Read the model definition and answer for the solid it produces. Units are mm, in the model's axes. Face numbers are marked on the shaded views. A direction names the side the tool comes from. Coordinates: 2 decimals unless noted, no trailing zeros. Loops run counter-clockwise (first coordinate to the right, second up) from the corner with the lowest first, then second, coordinate; pieces in that order, holes last. Notation, with made-up numbers: M -33.75,67.5 L -3.75,67.5 A12 ccw -3.75,75.5 Z; hole C 20,26 d11. An arc over 180 degrees is marked long. Put each result on its own line as item: value.
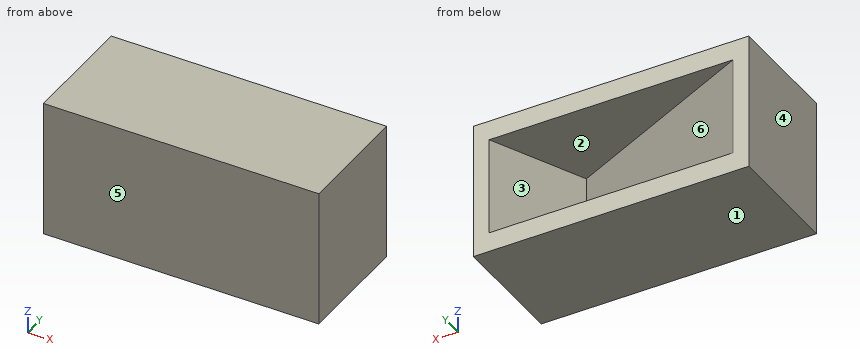
from build123d import *

# Parameters (mm, degrees)
SKETCH1_W           = 35
SKETCH1_H           = 17.5
BOSS_EXTRUDE2_DEPTH = 7.5
CUT_EXTRUDE2_DEPTH  = 6.25


with BuildPart() as part:
    # Sketch1 → Boss-Extrude2 (new, symmetric)
    with BuildSketch(Plane(origin=(0, 0, 0), x_dir=(1, 0, 0), z_dir=(0, 1, 0))):
        Rectangle(SKETCH1_W, SKETCH1_H)
    extrude(amount=BOSS_EXTRUDE2_DEPTH, both=True)

    # Sketch5 → Cut-Extrude2 (cut, symmetric)
    with BuildSketch(Plane.XY):
        Polygon((-15.5, 7.5), (9.96320795, -4.373688868), (15.5, 7.5), align=None)
    extrude(amount=CUT_EXTRUDE2_DEPTH, both=True, mode=Mode.SUBTRACT)


solid = part.part
1) Find section A-A, the plane y = 4.25. Write down the section's boundary in (x, z).
Answer list:
outline: M -17.5,-8.75 L 17.5,-8.75 L 17.5,8.75 L -17.5,8.75 Z; hole M -8.53,-6.25 L 13.98,-6.25 L 13.98,6.25 L -8.53,6.25 Z
2) Find section B-B, the plane x = -6. Write down the section's boundary in (y, z).
Answer list:
outline: M -7.5,-8.75 L 7.5,-8.75 L 7.5,-6.25 L 3.07,-6.25 L 3.07,6.25 L 7.5,6.25 L 7.5,8.75 L -7.5,8.75 Z
3) Find section D-D, the plane y = 2. Write down the section's boundary in (x, z).
Answer list:
outline: M -17.5,-8.75 L 17.5,-8.75 L 17.5,8.75 L -17.5,8.75 Z; hole M -3.71,-6.25 L 12.94,-6.25 L 12.94,6.25 L -3.71,6.25 Z
4) Find section C-C, the plane z = 1.5. Write down the section's boundary in (x, y), plus the area to 3 significant figures.
Answer list:
outline: M -17.5,-7.5 L 17.5,-7.5 L 17.5,7.5 L 15.5,7.5 L 9.96,-4.37 L -15.5,7.5 L -17.5,7.5 Z
area: 341 mm^2
5) Determine the mould class of the marked faces 1, 2, 3 and 4 for opening direction X: released by +X, released by -X, zero draft, split by the parting line, or undercut.
Answer list:
face 1: zero draft
face 2: undercut
face 3: undercut
face 4: released by -X
6) Which of the six approach directions +Z, -Z, +X, -X, +Y, -Y give full straight-line access (tool end or side, diameter ignored) to the marked faces 5 and 6?
Answer list:
face 5: +Z, -Z, +X, -X, -Y
face 6: +Y
7) Straight lines are drawn through the part: line 1 (Z direction, x = 8, y = -3.25); line 2 (X direction, y = 5.75, z = -1); line 3 (X direction, y = 1.5, z = -4). For each, find the intervals that lie inside material, in ascending order. Write a range as [from, to].
Answer list:
line 1: z = [-8.75, -6.25], [6.25, 8.75]
line 2: x = [-17.5, -11.75], [14.68, 17.5]
line 3: x = [-17.5, -2.63], [12.7, 17.5]
